Input: part model. Units: mm. Frame: model coordinates. Give positions to 0.01 mm unless a question says otherwise; leave off trailing zeros. Order: outer loops, then holes, each group sorted by start corner. A loop starts at its lowest first (then second) coordinate and runs counter-clockwise, first axis right, second up. Notation, with made-up numbers: (20, 79.5) -> (32, 79.5) arc R28 cw to (32, 102.5) -> close; hole circle Ø5 at (86.25, 45). An arc over 180 degrees is marked (long way). Use a Markdown table: item, result. Add a question column.
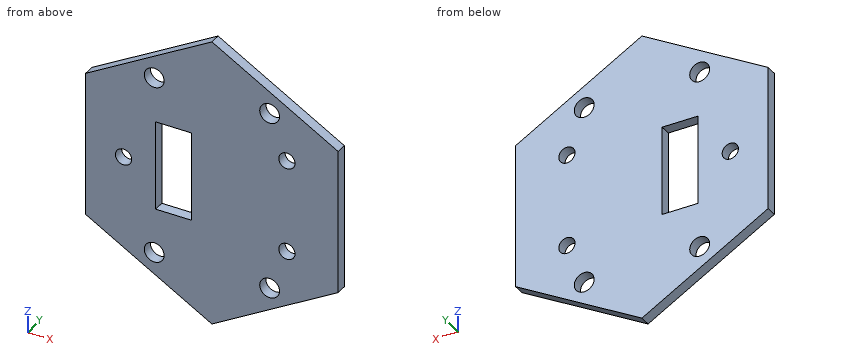
from build123d import *

# Parameters (mm, degrees)
SKETCH1_R           = 2.25
SKETCH1_R_2         = 2.75
SKETCH1_W           = 10
SKETCH1_H           = 25
BOSS_EXTRUDE1_DEPTH = 3


with BuildPart() as part:
    # Sketch1 → Boss-Extrude1 (new body)
    with BuildSketch(Plane(origin=(0, 0, 0), x_dir=(1, 0, 0), z_dir=(0, 1, 0))):
        Polygon((0, -40.414518843), (35, -20.207259422), (35, 20.207259422), (0, 40.414518843), (-35, 20.207259422), (-35, -20.207259422), align=None)
        with Locations(Location((20.792689758, 12.958165481, 0), (0, 0, 270))):
            Circle(SKETCH1_R, mode=Mode.SUBTRACT)
        with Locations(Location((20.794392615, -12.955432674, 0), (0, 0, 270))):
            Circle(SKETCH1_R, mode=Mode.SUBTRACT)
        with Locations(Location((-24.5, 0.406188596, 0), (0, 0, 270))):
            Circle(SKETCH1_R, mode=Mode.SUBTRACT)
        with Locations(Location((-16, 25, 0), (0, 0, 270))):
            Circle(SKETCH1_R_2, mode=Mode.SUBTRACT)
        with Locations(Location((16, 25, 0), (0, 0, 270))):
            Circle(SKETCH1_R_2, mode=Mode.SUBTRACT)
        with Locations(Location((-16, -25, 0), (0, 0, 270))):
            Circle(SKETCH1_R_2, mode=Mode.SUBTRACT)
        with Locations(Location((16, -25, 0), (0, 0, 270))):
            Circle(SKETCH1_R_2, mode=Mode.SUBTRACT)
        with Locations((-10.599366241, 0)):
            Rectangle(SKETCH1_W, SKETCH1_H, mode=Mode.SUBTRACT)
    extrude(amount=BOSS_EXTRUDE1_DEPTH)


solid = part.part
Q1. Section query B-B (z = -25). Return loops of the section in (x, y), plus the area to 3 significant figures.
Q2. First-contact query: pin 1 (3.5 mm diameter, centred on x = -16, z = 25, fed in from -Y); pin 2 (1.5 mm diameter, centred on x = -12, y = 1.5, fed in from +Z). Flat tips, straight axial feed; report the tip coordinate or a pass-through.
Q3. Ray query, line 1 (X direction, y = 2.35, z = 6.5); line 2 (X direction, y = 0.55, z = -12); line 3 (X direction, y = 0.75, z = -25). Return the intervals inside material, ascending.
Q4. Section query A-A (x = -25.5). Return loops of the section in (y, z), plus the area to 3 significant figures.
Q5. Section query C-C (z = 7.5). Return loops of the section in (x, y).
Q6. Section query D-D (y = 1.4). Give the number of separate pieces and of enclosed holes in the cut face, plus the area to 3 significant figures.
Solution:
| question | item | result |
|---|---|---|
| 1 | outline | (-26.7, 0) -> (-18.75, 0) -> (-18.75, 3) -> (-26.7, 3) -> close; (-13.25, 0) -> (13.25, 0) -> (13.25, 3) -> (-13.25, 3) -> close; (18.75, 0) -> (26.7, 0) -> (26.7, 3) -> (18.75, 3) -> close |
| 1 | area | 127 mm² |
| 2 | pin 1 | passes through |
| 2 | pin 2 | stops at z = 33.92 |
| 3 | line 1 | x = -35 to -15.6, -5.6 to 35 |
| 3 | line 2 | x = -35 to -15.6, -5.6 to 18.76, 22.83 to 35 |
| 3 | line 3 | x = -26.7 to -18.75, -13.25 to 13.25, 18.75 to 26.7 |
| 4 | outline | (0, -25.69) -> (3, -25.69) -> (3, -2.42) -> (0, -2.42) -> close; (0, 1.61) -> (3, 1.61) -> (3, 25.69) -> (0, 25.69) -> close |
| 4 | area | 142 mm² |
| 5 | outline | (-35, 0) -> (-15.6, 0) -> (-15.6, 3) -> (-35, 3) -> close; (-5.6, 0) -> (35, 0) -> (35, 3) -> (-5.6, 3) -> close |
| 6 | separate pieces | 1 |
| 6 | enclosed holes | 8 |
| 6 | area | 3,850 mm² |
